Could you check a few things on this drawing? It's one solid part, dimensions in mm from its lowest x, y, z. A direction names the side the tool comes from. Give positions to 0.01 mm unless a question says otherwise; leave off trailing zeros. Order: outer loops, then holes, each group sorted by start corner. A loop starts at its lowest first (then second) coordinate and runs counter-clockwise, first axis right, second up. Notation, with made-up numbers: (-24.75, 29) - (-4.75, 29) arc R31 cw to (-4.75, 57) - close; hole circle Ø10 at (-38, 12). An arc over 180 degrees is marked (long way). One line per question, with ' | ' between items. Start each with the question number.
1. Imagine slicing it at B-B (z = 2.75). Please give me the cut outline in (x, y), and give its area (3 significant figures).
2. Imagine slicing it at A-A (x = 44). Please give me the cut outline in (y, z).
3. Imagine slicing it at C-C (x = 26.5). Please give me the cut outline in (y, z).
4. I need wall thicknesses on probe 1 along X at (y, z) = (1.2, 15); probe 2 along X at (y, z) = (1.8, 27); probe 3 along X at (y, z) = (3.05, 13.75). Which ranges of each line are inside material? Lowest first, please. Write a range as from..to.
5. If we mould it in two halves opening along X, with no side actions, what happens to the marked faces 4, 5, 6 and 7? For each: released by +X, released by -X, zero draft, split by the parting line, or undercut.
6. Which directions (+Z, -Z, +X, -X, +Y, -Y) give clear straight access to the entire face, cutting with the end or side of a thin tool? Please do the marked faces 1, 2 and 3.
7. For P1, Ø1, axis at x = 28, y = 3.5, coming from the -Z side; P2, Ø1.5, axis at y = 3.5, z = 2, coming from the +X side, each with a flat end and sliding along its axis, tell me the tip position at first contact or that it passes through.
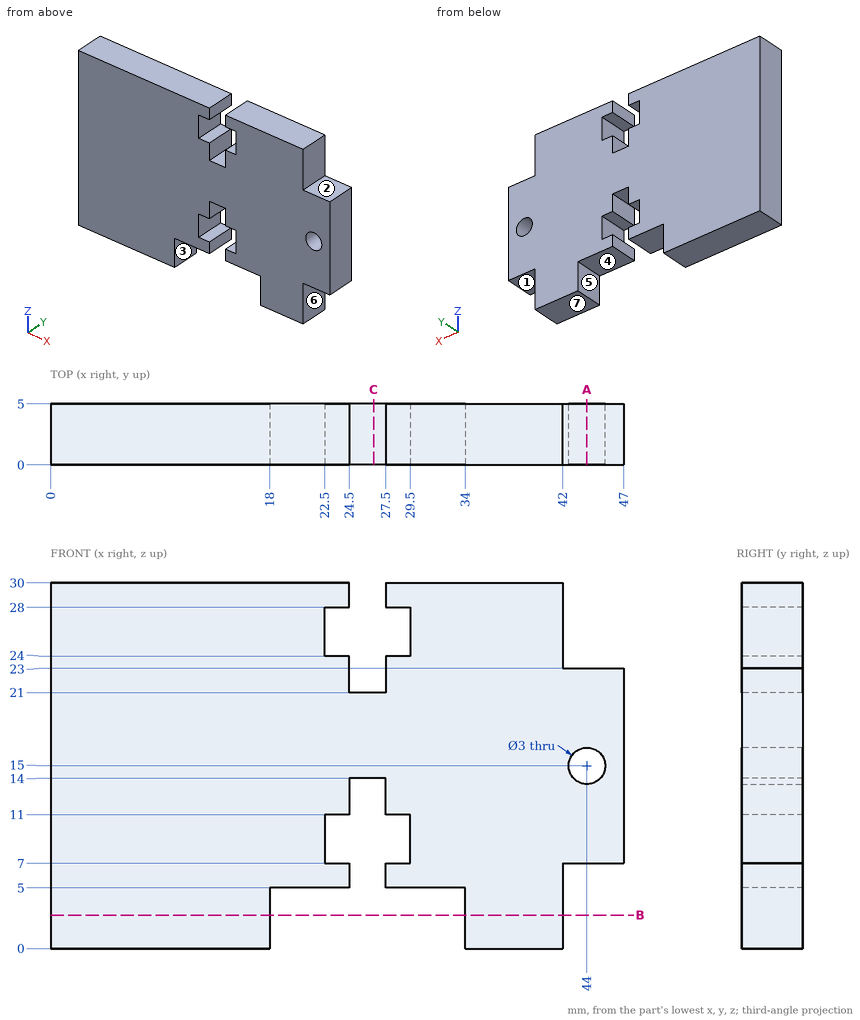
Results found:
1) outline: (0, 0) - (18, 0) - (18, 5) - (0, 5) - close; (34, 0) - (42, 0) - (42, 5) - (34, 5) - close | area: 130 mm2
2) outline: (0, 7) - (5, 7) - (5, 13.5) - (0, 13.5) - close; (0, 16.5) - (5, 16.5) - (5, 23) - (0, 23) - close
3) outline: (0, 14) - (5, 14) - (5, 21) - (0, 21) - close
4) probe 1: x = 0..42.5, 45.5..47 | probe 2: x = 0..22.5, 29.5..42 | probe 3: x = 0..24.5, 27.5..43.17, 44.83..47
5) face 4: undercut | face 5: undercut | face 6: released by +X | face 7: zero draft
6) face 1: -Z, +X, +Y, -Y | face 2: +Z, +X, +Y, -Y | face 3: -Z, +Y, -Y
7) P1: stops at z = 5 | P2: stops at x = 42
